Geometry: final body of the model. Coordinates: model frame, mm. A direction names the side the tool comes from. Round coordinates to 2 decimals unless told otherwise and drop trailing zeros. Loops run counter-clockwise (first coordinate to the right, second up) from the corner with the lowest first, then second, coordinate; pieces in that order, holes last. Notation, with made-up numbers: (-31.5, -13.75) - (-22.5, -13.75) arc R31 ccw to (-22.5, 24.25) - close; hole circle Ø2 at (81, 75.5). An arc over 180 degrees is marked (long way). Answer in a Markdown table with one row per item. Add a question column.
from build123d import *

# Parameters (mm, degrees)
F0_R      = 1.75
F1_DEPTH  = 10
F2_R      = 1.7838032989
F2_R_2    = 1.6991644828
F3_DEPTH  = 25
F5_W      = 23.6940248869
F5_H      = 47.8357747197
F6_DEPTH  = 25
F7_R      = 1.75
F8_DEPTH  = 10
F9_W      = 4.2999079451
F9_H      = 6.339606829
F9_W_2    = 3.9691450074
F9_H_2    = 1.433301717
F9_H_3    = 1.4884294942
F10_DEPTH = 25
F12_DEPTH = 10
F13_W     = 28.7822000682
F13_H     = 4.495148547
F14_DEPTH = 25
F16_DEPTH = 25
F17_R     = 3.5044645389
F17_R_2   = 3.3871652345
F18_DEPTH = 0.9


with BuildPart() as f1:
    # F0 (on Top) → F1 (new body)
    with BuildSketch(Plane.XY):
        with BuildLine():
            Line((8.2999998219, -21.1999956518), (8.2999998219, 21.2139172642))
            Line((8.2999998219, 21.2139172642), (-6.2000001781, 21.2139172642))
            Line((-6.2000001781, 21.2139172642), (-6.2000001781, 5.0756316632))
            Line((-6.2000001781, 5.0756316632), (-1.7000001781, 5.0756316632))
            ThreePointArc((-1.7000001781, 5.0756316632), (3.9999996856, -0.6243682004), (-1.7000001781, -6.3243680641))
            Line((-1.7000001781, -6.3243680641), (-6.2000001781, -6.3243680641))
            Line((-6.2000001781, -6.3243680641), (-6.2000001781, -21.1999956518))
            Line((-6.2000001781, -21.1999956518), (8.2999998219, -21.1999956518))
        make_face()
        with Locations((5.3999998219, -9.2503995063)):
            Circle(F0_R, mode=Mode.SUBTRACT)
    extrude(amount=F1_DEPTH)

    # F2 (on face) → F3 (cut)
    with BuildSketch(Plane.YZ.offset(8.2999998219)):
        with Locations((-17.2935956518, 5)):
            Circle(F2_R)
        with Locations((16.0253872642, 5)):
            Circle(F2_R_2)
    extrude(amount=-F3_DEPTH, mode=Mode.SUBTRACT)

    # F4: F1 across face


with BuildPart() as f1_1:
    add(f1.part)
    add(f1.part.mirror(Plane(origin=(-6.2000001781, 12.9732327122, 5), x_dir=(0, -1, 0), z_dir=(-1, 0, 0))))

    # F5 (on face) → F6 (cut)
    with BuildSketch(Plane.XY.offset(10)):
        with Locations((5.6470122654, 2.717891708)):
            Rectangle(F5_W, F5_H)
    extrude(amount=-F6_DEPTH, mode=Mode.SUBTRACT)

    # F7 (on face) → F8 (join, through all)
    with BuildSketch(Plane.XY.offset(10)):
        with Locations((-17.8000001781, -9.2503995063)):
            Circle(F7_R)
    extrude(amount=-F8_DEPTH)

    # F9 (on face) → F10 (cut)
    with BuildSketch(Plane.XY.offset(10)):
        with Locations((-11.4986333065, -10.246865917)):
            Rectangle(F9_W, F9_H)
        with Locations((-17.6728586666, -6.360411644)):
            Rectangle(F9_W_2, F9_H_2)
        with Locations((-17.6728586666, -14.1608840786)):
            Rectangle(F9_W_2, F9_H_3)
        with Locations((-11.0412049107, 9.0499585494)):
            Rectangle(F9_W, F9_H)
        with Locations((-17.2154302709, 12.9364128225)):
            Rectangle(F9_W_2, F9_H_2)
        with Locations((-17.2154302709, 5.1359403878)):
            Rectangle(F9_W_2, F9_H_3)
    extrude(amount=-F10_DEPTH, mode=Mode.SUBTRACT)

    # F11 (on face) → F12 (join, through all)
    with BuildSketch(Plane.XY.offset(10)):
        with BuildLine():
            Line((-10.7000001781, 3.9756317079), (-6.2000001781, 3.9756317079))
            Line((-6.2000001781, 3.9756317079), (-6.2000001781, 5.0756316632))
            Line((-6.2000001781, 5.0756316632), (-10.7000001781, 5.0756316632))
            ThreePointArc((-10.7000001781, 5.0756316632), (-16.4000000417, -0.6243682004), (-10.7000001781, -6.3243680641))
            Line((-10.7000001781, -6.3243680641), (-6.2000001781, -6.3243680641))
            Line((-6.2000001781, -6.3243680641), (-6.2000001781, -5.2243681088))
            Line((-6.2000001781, -5.2243681088), (-10.7000001781, -5.2243681088))
            ThreePointArc((-10.7000001781, -5.2243681088), (-15.3000000864, -0.6243682004), (-10.7000001781, 3.9756317079))
        make_face()
    extrude(amount=-F12_DEPTH)

    # F13 (on face) → F14 (cut)
    with BuildSketch(Plane(origin=(-20.7000001781, 0, 0), x_dir=(0, -1, 0), z_dir=(-1, 0, 0))):
        with Locations((0.6876317784, 2.2475742735)):
            Rectangle(F13_W, F13_H)
    extrude(amount=-F14_DEPTH, mode=Mode.SUBTRACT)

    # F15 (on face) → F16 (cut)
    with BuildSketch(Plane.XY.offset(10)):
        with BuildLine():
            Line((-14.0170669183, -4.8394002952), (-10.3995706886, -4.8394002952))
            Line((-10.3995706886, -4.8394002952), (-10.3995706886, 3.5300727468))
            Line((-10.3995706886, 3.5300727468), (-14.0170669183, 3.5300727468))
            ThreePointArc((-14.0170669183, 3.5300727468), (-16.5291727201, -0.6546637742), (-14.0170669183, -4.8394002952))
        make_face()
    extrude(amount=-F16_DEPTH, mode=Mode.SUBTRACT)

    # F17 (on face) → F18 (cut)
    with BuildSketch(Plane(origin=(-20.7000001781, 0, 0), x_dir=(0, -1, 0), z_dir=(-1, 0, 0))):
        with Locations((-16.0253872642, 5)):
            Circle(F17_R)
        with Locations((17.2935956518, 5)):
            Circle(F17_R_2)
    extrude(amount=-F18_DEPTH, mode=Mode.SUBTRACT)


solid = f1_1.part
1) Section D-D, the plane y = -8. Return the cut outline in (x, z).
2) Material intervals for line 1 along Y through (x, z) = (-9, 8.75); line 2 along X through (y, z) = (11.5, 7.75); line 3 along Y through (x, z) = (-9, 5), sorted ascending. Write a range as from..to.
3) Reachability of faces 1 (the flat face through (-13, -4.839, 7)), 2 (the flat face through (-19.8, 18, 4)), 3 (the flat face through (-11, 5.88, 7)) from +Z, -Z, +X, -X, +Y, -Y: full face, straight path, thin tool, end or side. Return the list, or none.
4) Section A-A, the plane x = -18.5. Return the cut outline in (y, z), and give its area (3 significant figures).
5) Contact query for a flat-ended pin moving along its axis: pin 1 Ø4 at (x, y) = (-16.5, -3.5) entering from -Z. Output: stop coordinate, or through.
6) Section C-C, the plane x = -10. Return the cut outline in (y, z).
7) Section B-B, the plane z = 0.75. Return the cut outline in (x, y), and give its area (3 significant figures).
8) Pull-direction query (X, two-part tool) for faces 4 (the flat face through (-17, 0, 4.495)), 5 (the cylindrical face through (-11.63, -5.13, 7.29)), 6 (the flat face through (-17, 4.392, 7)); classes: pulls with the +X half, pulls with the -X half, needs draft (parallel to the pull), parting line crosses it, or undercut.
Evaluation:
| question | item | result |
|---|---|---|
| 1 | outline | (-20.7, 4.5) - (-13.65, 4.5) - (-13.65, 10) - (-20.7, 10) - close; (-9.35, 4.5) - (-6.2, 4.5) - (-6.2, 10) - (-9.35, 10) - close |
| 2 | line 1 | y = -21.2..-5.22, 3.98..5.88, 12.22..21.21 |
| 2 | line 2 | x = -20.7..-13.19, -8.89..-6.2 |
| 2 | line 3 | y = -21.2..-19.08, -15.51..-5.22, 3.98..5.88, 12.22..14.33, 17.72..21.21 |
| 3 | face 1 | +Z, -Z, +X |
| 3 | face 2 | -X |
| 3 | face 3 | +Z, -Z |
| 4 | outline | (-21.2, 0) - (-15.08, 0) - (-15.08, 4.5) - (-14.91, 4.5) - (-14.91, 10) - (-21.2, 10) - close; (-13.42, 4.5) - (-7.08, 4.5) - (-7.08, 10) - (-13.42, 10) - close; (-5.64, 4.5) - (4.39, 4.5) - (4.39, 10) - (-5.64, 10) - close; (5.88, 4.5) - (12.22, 4.5) - (12.22, 10) - (5.88, 10) - close; (13.65, 4.5) - (13.7, 4.5) - (13.7, 0) - (21.21, 0) - (21.21, 10) - (13.65, 10) - close; hole circle Ø3.57 at (-17.29, 5); hole circle Ø3.4 at (16.03, 5) |
| 4 | area | 244 mm² |
| 5 | pin 1 | stops at z = 4.5 |
| 6 | outline | (-21.2, 0) - (-15.08, 0) - (-15.08, 4.5) - (-13.42, 4.5) - (-13.42, 10) - (-21.2, 10) - close; (-7.08, 4.5) - (-5.22, 4.5) - (-5.22, 10) - (-7.08, 10) - close; (3.98, 4.5) - (5.88, 4.5) - (5.88, 10) - (3.98, 10) - close; (12.22, 4.5) - (13.7, 4.5) - (13.7, 0) - (21.21, 0) - (21.21, 10) - (12.22, 10) - close; hole circle Ø3.57 at (-17.29, 5); hole circle Ø3.4 at (16.03, 5) |
| 7 | outline | (-20.7, -21.2) - (-6.2, -21.2) - (-6.2, -15.08) - (-20.7, -15.08) - close; (-20.7, 13.7) - (-6.2, 13.7) - (-6.2, 21.21) - (-20.7, 21.21) - close |
| 7 | area | 198 mm² |
| 8 | face 4 | needs draft |
| 8 | face 5 | pulls with the +X half |
| 8 | face 6 | undercut |
